Could you check a few things on this drawing? It's one solid part, dimensions in mm from its lowest x, y, z. Give positions to 0.01 mm unless a question says otherwise; leave off trailing zeros. Order: outer loops, then holes, each group sorted by start corner. A loop starts at its lowest first (then second) coordinate and runs counter-clockwise, first axis right, second up. Notation, with made-up numbers: (63.25, 81.5) - (121.25, 81.5) arc R17 ccw to (121.25, 110.5) - close; hole circle Ø11 at (78.5, 86.25). An arc over 180 degrees is marked (long way). Return JSON: item names as keys, results as strings.
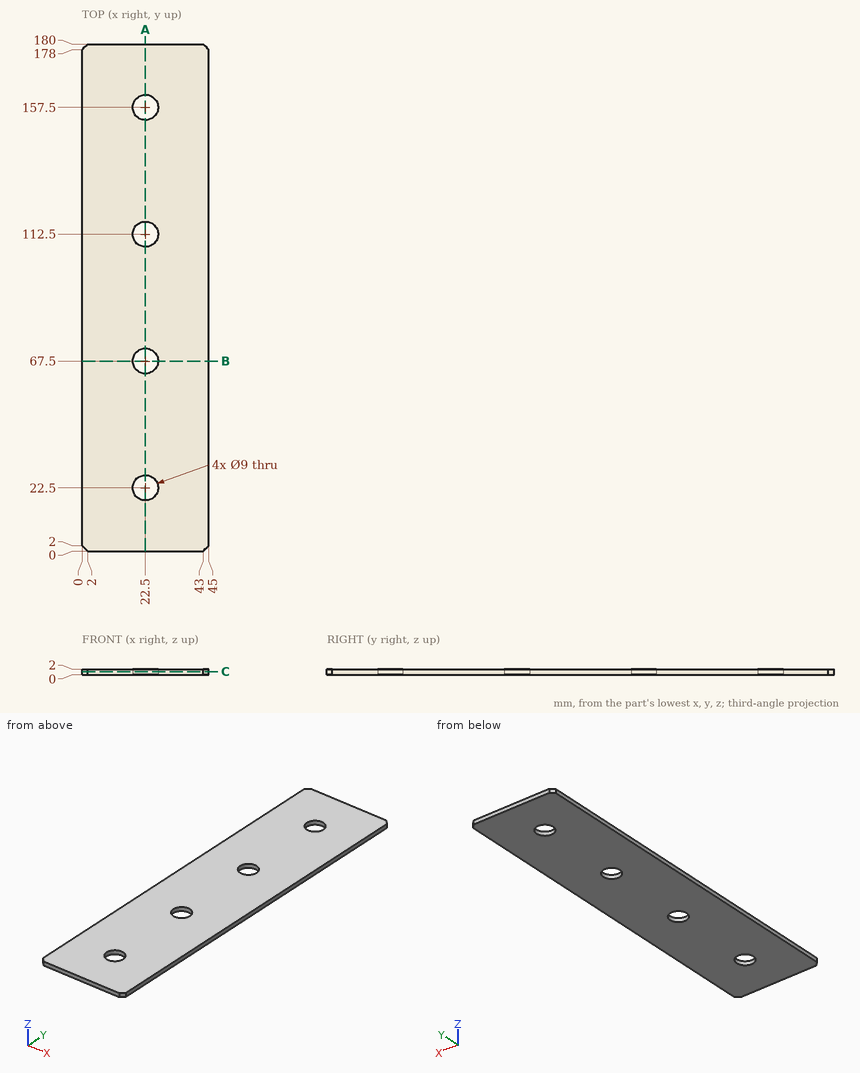
1. If I drill on L1, parallel to Y at x = 22, z = 0.7; L2, parallel to X at y = 109.5, z = 1.5; L3, parallel to Y at x = 43.5, z = 1.9, over which ranges is the centre line in solid material (lowest first)? Write a range as [from, to].
Checks:
{"L1": "[0, 18.03], [26.97, 63.03], [71.97, 108.03], [116.97, 153.03], [161.97, 180]", "L2": "[0, 19.15], [25.85, 45]", "L3": "[0.5, 179.5]"}
2. Suppose I cut it at C-C (z = 1.1). List the corners of the cut face in (x, y) for me, plus the area to 3 significant figures.
Checks:
{"outline": "(0, 2) - (2, 0) - (43, 0) - (45, 2) - (45, 178) - (43, 180) - (2, 180) - (0, 178) - close; hole circle Ø9 at (22.5, 22.5); hole circle Ø9 at (22.5, 67.5); hole circle Ø9 at (22.5, 112.5); hole circle Ø9 at (22.5, 157.5)", "area": "7,840 mm^2"}
3. Suppose I cut it at B-B (y = 67.5). List the corners of the cut face in (x, z) for me, plus the area to 3 significant figures.
Checks:
{"outline": "(0, 0) - (18, 0) - (18, 2) - (0, 2) - close; (27, 0) - (45, 0) - (45, 2) - (27, 2) - close", "area": "72.0 mm^2"}
4. For pin 1 Ø7 at (x, y) = (22.5, 112.5) entering from +Z, with a flat end and sliding along its axis, tell me the tip position at first contact or that it passes through.
Checks:
{"pin 1": "through"}
5. Suppose I cut it at A-A (x = 22.5). List the corners of the cut face in (y, z) for me, plus the area to 3 significant figures.
Checks:
{"outline": "(0, 0) - (18, 0) - (18, 2) - (0, 2) - close; (27, 0) - (63, 0) - (63, 2) - (27, 2) - close; (72, 0) - (108, 0) - (108, 2) - (72, 2) - close; (117, 0) - (153, 0) - (153, 2) - (117, 2) - close; (162, 0) - (180, 0) - (180, 2) - (162, 2) - close", "area": "288 mm^2"}
